Design review of the part shown in the three views and the two pictorial views. Dimensions are in mm from the part's minimum x, y and z. A direction names the side the tool comes from. Round coordinates to 2 decimals unless told otherwise and drop trailing zeros. Write each loop counter-clockwise with the first axis right and the second up, starting at its lowest first coordinate (ties: lowest second). Pieces come first, ordered by that corner, then holes. Notation, with made-up numbers: (-33.5, -6.75) - (1.5, -6.75) arc R5 cw to (1.5, 2.25) - close; hole circle Ø1 at (56.25, 56.5). An arc over 180 degrees is marked (long way). Use one line per item in the form item = value.
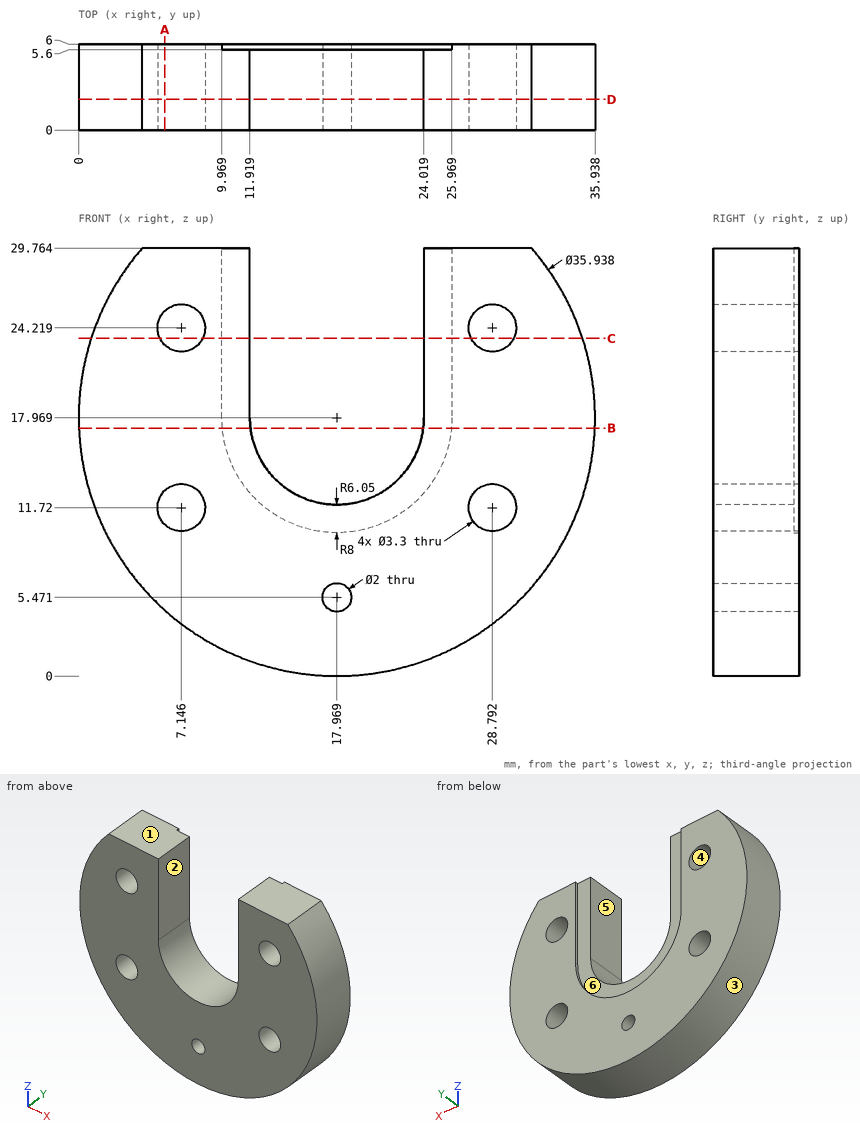
(1) The part is to be moulded in two halves that separate along X. For the marked faces 1, 2 and 3, say which applies: +X half, -X half, draft (parallel to the pull), parting line (faces both ways), or undercut.
Geometry results:
face_1 = draft
face_2 = undercut
face_3 = parting line
(2) Insertion check: P1, Ø2, axis at y = 4, z = 12, coming from the +X side. The pin has a flat end and moves straight along its axis. Give the tip position at first contact, or say it passes through.
Geometry results:
P1 = 35.24
(3) Add section D-D on y = 2.15. Count the separate pieces of the cut face and the enclosed holes in it, then the cut area to 3 significant figures.
Geometry results:
separate_pieces = 1
enclosed_holes = 5
area = 661 mm2
(4) Add section C-C on z = 23.5. Write out the cut boundary in (x, y).
Geometry results:
outline = (0.87, 0) - (5.66, 0) - (5.66, 6) - (0.87, 6) - close; (8.63, 0) - (11.92, 0) - (11.92, 5.6) - (9.97, 5.6) - (9.97, 6) - (8.63, 6) - close; (24.02, 0) - (27.31, 0) - (27.31, 6) - (25.97, 6) - (25.97, 5.6) - (24.02, 5.6) - close; (30.28, 0) - (35.07, 0) - (35.07, 6) - (30.28, 6) - close
(5) Add section A-A on x = 6. Write out the cut boundary in (y, z) (1 decimal).
Geometry results:
outline = (0, 4.6) - (6, 4.6) - (6, 10.5) - (0, 10.5) - close; (0, 12.9) - (6, 12.9) - (6, 23) - (0, 23) - close; (0, 25.4) - (6, 25.4) - (6, 29.8) - (0, 29.8) - close
(6) To check wall thickness, follow L1, parallel to Z at x = 28.5, y = 2.7 (1 decimal); L2, parallel to Z at x = 8, y = 3.8 (1 decimal); L3, parallel to X at y = 4.8, z = 11.25 (1 decimal). State the ranges of each line that lie inside material, in increasing order.
Geometry results:
L1 = 3.4 to 10.1, 13.3 to 22.6, 25.8 to 29.8
L2 = 3 to 10.3, 13.1 to 22.8, 25.6 to 29.8
L3 = 1.3 to 5.6, 8.7 to 27.2, 30.4 to 34.6
(7) Machinability: for the marked faces 4, 5 and 6, which of the approach directions +Z, -Z, +X, -X, +Y, -Y give a long, thin tool a straight path to every point of the face, cutting with its end or side? Answer none if there is none.
Geometry results:
face_4 = +Y, -Y
face_5 = +Z, +Y, -Y
face_6 = +Z, +Y
(8) Add section B-B on z = 17.25. Write out the cut boundary in (x, y) (1 decimal).
Geometry results:
outline = (0, 0) - (12, 0) - (12, 5.6) - (10, 5.6) - (10, 6) - (0, 6) - close; (24, 0) - (35.9, 0) - (35.9, 6) - (25.9, 6) - (25.9, 5.6) - (24, 5.6) - close
